Part model, mm, in its own coordinate system. A direction names the side the tool comes from. Coordinates: 2 decimals unless noted, no trailing zeros. Loops run counter-clockwise (first coordinate to the right, second up) from the corner with the lowest first, then second, coordinate; pieces in that order, holes last. Notation, with made-up numbers: (-36.5, -32.75) - (-0.5, -32.75) arc R21 cw to (-0.5, -16.75) - close; hole circle Ø7 at (-15.75, -17.75). An arc over 180 degrees is marked (long way). Use a Markdown table: item, result. Add a question column.
1. Pull direction Z, two halves, no side cores. Call faces 6 (the flat face through (-67, 18, 12)), 7 (the cylindrical face through (-42.157, 10.681, 8.193)), 8 (the cylindrical face through (14, 5, 0)): pulls with the +Z half, pulls with the -Z half, needs draft (parallel to the pull), parting line crosses it, or undercut.
2. Drop flat-ended pins along their axis: pin 1 (3.5 mm diameter, centred on x = 0, z = 15.5, fed in from +Y); pin 2 (10 mm diameter, centred on y = 28.5, z = -9, fed in from +X); pin 3 (0.9 mm diameter, centred on x = -0.5, z = 16, fed in from -Y). Give the stop position or say it passes through.
3. Band-saw the part on B-B, the plane y = 20. Give the cut face in (x, z), plus the area to 3 significant figures.
4. Band-saw the part on C-C, the plane z = -5. Give the cut face in (x, y).
5. Band-saw the part on D-D, the plane x = 3. Give the cut face in (y, z).
6. Wall check: probe 1 along Z at (x, y) = (0, 7.5); probe 2 along Z at (x, y) = (-15.5, 4.25); probe 3 along Y at (x, z) = (47.5, 12). Give the ranges that are in metal, low to high. Write a range as [from, to].
7. Band-saw the part on A-A, the plane z = 12. Give the cut face in (x, y).
8. 3-axis set-ups, long thin cutter, end or side, ignore diameter. For faces 1 (the cylindrical face through (0, 17, -18)), 2 (the flat face through (67, 18, 12)), 3 (the cylindrical face through (4.57, 40.902, -7.167)), 4 (the cylindrical face through (-17, 5, 0)), 5 (the cylindrical face through (42.157, 10.681, 8.193)): which of +Z, -Z, +X, -X, +Y, -Y reach the whole face in a straight line?
from build123d import *

# Parameters (mm, degrees)
SKETCH1_R                = 8.5
SKETCH1_R_2              = 7
BOSS_EXTRUDE1_DEPTH      = 48
SKETCH2_R                = 8.5
BOSS_EXTRUDE2_DEPTH      = 34
SKETCH3_R                = 1.5
CUT_EXTRUDE1_DEPTH       = 10
SKETCH4_R                = 8.25
BOSS_EXTRUDE3_DEPTH      = 67
BOSS_EXTRUDE3_DEPTH_BACK = 67


with BuildPart() as part:
    # Sketch1 → Boss-Extrude1 (new body)
    with BuildSketch(Plane(origin=(0, 0, 0), x_dir=(1, 0, 0), z_dir=(0, 1, 0))):
        Circle(SKETCH1_R)
        Circle(SKETCH1_R_2, mode=Mode.SUBTRACT)
    extrude(amount=BOSS_EXTRUDE1_DEPTH)

    # Sketch2 → Boss-Extrude2 (add)
    with BuildSketch(Plane.XZ):
        with BuildLine():
            Line((-18, 22), (18, 22))
            Line((18, 22), (18, 0))
            ThreePointArc((18, 0), (0, -18), (-18, 0))
            Line((-18, 0), (-18, 22))
        make_face()
        Circle(SKETCH2_R, mode=Mode.SUBTRACT)
    extrude(amount=-BOSS_EXTRUDE2_DEPTH)

    # Sketch3 → Cut-Extrude1 (cut)
    with BuildSketch(Plane.XZ):
        with Locations((0, -15.5)):
            Circle(SKETCH3_R)
        with Locations((-15.5, 0)):
            Circle(SKETCH3_R)
        with Locations((0, 15.5)):
            Circle(SKETCH3_R)
        with Locations((15.5, 0)):
            Circle(SKETCH3_R)
    extrude(amount=-CUT_EXTRUDE1_DEPTH, mode=Mode.SUBTRACT)

    # Sketch4 → Boss-Extrude3 (add, two sides)
    with BuildSketch(Plane(origin=(0, 0, 0), x_dir=(0, 0, -1), z_dir=(1, 0, 0))) as boss_extrude3_sk:
        with Locations((-12, 18)):
            Circle(SKETCH4_R)
    extrude(amount=BOSS_EXTRUDE3_DEPTH)
    extrude(boss_extrude3_sk.sketch, amount=-BOSS_EXTRUDE3_DEPTH_BACK)


solid = part.part
Geometry check:
| question | item | result |
|---|---|---|
| 1 | face 6 | needs draft |
| 1 | face 7 | parting line crosses it |
| 1 | face 8 | undercut |
| 2 | pin 1 | stops at y = 34 |
| 2 | pin 2 | stops at x = 17.55 |
| 2 | pin 3 | stops at y = 10 |
| 3 | outline | (-67, 4) - (-18, 4) - (-18, 0) arc R18 ccw to (18, 0) - (18, 4) - (67, 4) - (67, 20) - (18, 20) - (18, 22) - (-18, 22) - (-18, 20) - (-67, 20) - close; hole (-5.75, 4) arc R7 ccw (long way) to (5.75, 4) - close |
| 3 | area | 2,740 mm^2 |
| 4 | outline | (-17.29, 0) - (-4.9, 0) - (-4.9, 48) - (-6.87, 48) - (-6.87, 34) - (-17.29, 34) - close; (4.9, 0) - (17.29, 0) - (17.29, 34) - (6.87, 34) - (6.87, 48) - (4.9, 48) - close |
| 5 | outline | (0, -17.75) - (34, -17.75) - (34, -7.95) - (48, -7.95) - (48, -6.32) - (0, -6.32) - close; (0, 6.32) - (12.01, 6.32) arc R8.25 ccw to (23.99, 6.32) - (48, 6.32) - (48, 7.95) - (34, 7.95) - (34, 22) - (0, 22) - close |
| 6 | probe 1 | z = [-18, -17], [-14, -7], [7, 14], [17, 22] |
| 6 | probe 2 | z = [-9.15, -1.5], [1.5, 22] |
| 6 | probe 3 | y = [9.75, 26.25] |
| 7 | outline | (-67, 9.75) - (-18, 9.75) - (-18, 0) - (18, 0) - (18, 9.75) - (67, 9.75) - (67, 26.25) - (18, 26.25) - (18, 34) - (-18, 34) - (-18, 26.25) - (-67, 26.25) - close |
| 8 | face 1 | -Z, +Y, -Y |
| 8 | face 2 | +Z, -Z, +X, +Y, -Y |
| 8 | face 3 | +Y |
| 8 | face 4 | -Y |
| 8 | face 5 | +X |
